CAD build for the part. Positions are in the model's coordinates, mm. A direction names the side the tool comes from. Round coordinates to 2 decimals unless told otherwise and drop trailing zeros. Write each loop counter-clockwise with the first axis right and the second up, starting at its lowest first coordinate (ties: lowest second). Pieces come first, ordered by that corner, then holes. Notation, with made-up numbers: (-27, -21.5) - (13, -21.5) arc R17 cw to (13, -6.5) - close; hole circle Ø8 at (27.5, -35.75). An arc over 180 degrees is marked (long way). Use one line per item in the form item = value. Start each with the question number.
Item 1: Band-saw the part on A-A, the plane z = 0. List the corners of the cut face in (x, y) (3 decimals), and give its area (3 significant figures).
Item 2: Band-saw the part on C-C, the plane x = 13.25. List the corners of the cut face in (y, z), and give its area (3 significant figures).
Item 3: Drill centre lines: L1, parallel to Y at x = 4.5, z = 0 (3 decimals); L2, parallel to X at y = -23, z = 6; L3, parallel to Z at x = 8.75, y = -6. Where is each one in solid material? Low to high.
Item 4: Pull direction Z, two halves, no side cores. Call faces 4 (the flat face through (14, -3, -3)), 5 (the flat face through (11.5, -3, -3)), 6 (the cylindrical face through (12.768, -3.905, 0.867)), 7 (the cylindrical face through (8.93, -6.32, -15.24)): +Z half, -Z half, draft (parallel to the pull), parting line (faces both ways), or undercut.
Item 5: Band-saw the part on D-D, the plane x = 6.25. List the corners of the cut face in (y, z) (3 decimals), and give its area (3 significant figures).
Item 6: Tool access for faces 1 (the cylindrical face through (1.26, 13.24, 13.35)), 2 (the flat face through (4, 0, 17)), 3 (the cylindrical face through (5.67, 3.94, 12.52)): list every direction of +Z, -Z, +X, -X, +Y, -Y with a clear straight run to the whole face (end or side of a thin tool).
Item 7: Pin check, flat tips, straight feed: pin 1 (4.5 mm diameter, centred on y = -14.5, z = -14.5, fed in from +X); pin 2 (5 mm diameter, centred on x = 11, y = -9, fed in from +Z); pin 3 (2 mm diameter, centred on x = 9.5, y = 13, fed in from -Z). Stop position of each tip, or through.
Item 8: Band-saw the part on B-B, the plane y = 0. List the corners of the cut face in (x, z) (3 decimals).
from build123d import *

# Parameters (mm, degrees)
SKETCH1_R                                       = 25
BOSS_EXTRUDE1_DEPTH                             = 4
SKETCH2_R                                       = 16.5
BOSS_EXTRUDE2_DEPTH                             = 10
SKETCH3_R                                       = 12.5
CUT_EXTRUDE1_DEPTH                              = 11.5
SKETCH4_R                                       = 4
CUT_EXTRUDE2_DEPTH                              = 4
M3_CLEARANCE_HOLE1_D                            = 3.4
M3_CLEARANCE_HOLE1_DEPTH                        = 10
CSK_FOR_M3_FLAT_HEAD_MACHINE_SCREW1_D           = 3.4
CSK_FOR_M3_FLAT_HEAD_MACHINE_SCREW1_CSINK_D     = 6.3
CSK_FOR_M3_FLAT_HEAD_MACHINE_SCREW1_CSINK_ANGLE = 90
CIRPATTERN1_COUNT                               = 4
SKETCH10_R                                      = 13.125
CUT_EXTRUDE3_DEPTH                              = 11.5


with BuildPart() as part:
    # Sketch1 → Boss-Extrude1 (new body)
    with BuildSketch(Plane(origin=(0, 0, 0), x_dir=(0, 0, -1), z_dir=(1, 0, 0))):
        Circle(SKETCH1_R)
    extrude(amount=BOSS_EXTRUDE1_DEPTH)

    # Sketch2 → Boss-Extrude2 (add)
    with BuildSketch(Plane(origin=(4, 0, 0), x_dir=(0, 0, -1), z_dir=(1, 0, 0))):
        Circle(SKETCH2_R)
    extrude(amount=BOSS_EXTRUDE2_DEPTH)

    # Sketch3 → Cut-Extrude1 (cut)
    with BuildSketch(Plane.ZY):
        Circle(SKETCH3_R)
    extrude(amount=-CUT_EXTRUDE1_DEPTH, mode=Mode.SUBTRACT)

    # Sketch4 → Cut-Extrude2 (cut)
    with BuildSketch(Plane(origin=(14, 0, 0), x_dir=(0, 0, -1), z_dir=(1, 0, 0))):
        Circle(SKETCH4_R)
    extrude(amount=-CUT_EXTRUDE2_DEPTH, mode=Mode.SUBTRACT)

    # M3 Clearance Hole1
    with Locations(Plane(origin=(14, 0, 0), x_dir=(0, 0, -1), z_dir=(1, 0, 0))):
        with Locations((8.5, 0), (-8.5, 0)):
            Hole(M3_CLEARANCE_HOLE1_D / 2, depth=M3_CLEARANCE_HOLE1_DEPTH)

    # CSK for M3 Flat Head Machine Screw1 (through all)
    with Locations(Plane(origin=(4, 0, 0), x_dir=(0, 0, -1), z_dir=(1, 0, 0))):
        with Locations((-14.495689014, -14.495689014)):
            csk_for_m3_flat_head_machine_screw1 = CounterSinkHole(CSK_FOR_M3_FLAT_HEAD_MACHINE_SCREW1_D / 2, CSK_FOR_M3_FLAT_HEAD_MACHINE_SCREW1_CSINK_D / 2, counter_sink_angle=CSK_FOR_M3_FLAT_HEAD_MACHINE_SCREW1_CSINK_ANGLE)

    # CirPattern1: CSK for M3 Flat Head Machine Screw1 ×4 about axis
    cirpattern1_axis = Axis((0, 0, 0), (1, 0, 0))
    for i in range(1, CIRPATTERN1_COUNT):
        add(csk_for_m3_flat_head_machine_screw1.rotate(cirpattern1_axis, i * 360 / CIRPATTERN1_COUNT), mode=Mode.SUBTRACT)

    # Sketch10 → Cut-Extrude3 (cut)
    with BuildSketch(Plane.ZY):
        Circle(SKETCH10_R)
    extrude(amount=-CUT_EXTRUDE3_DEPTH, mode=Mode.SUBTRACT)


solid = part.part
Determined:
q1.outline = (0, -25) - (4, -25) - (4, -16.5) - (14, -16.5) - (14, -4) - (11.5, -4) - (11.5, -13.125) - (0, -13.125) - close; (0, 13.125) - (11.5, 13.125) - (11.5, 4) - (14, 4) - (14, 16.5) - (4, 16.5) - (4, 25) - (0, 25) - close
q1.area = 208 mm²
q2.outline = circle Ø33 at (0, 0); hole circle Ø8 at (0, 0); hole circle Ø3.4 at (0, -8.5); hole circle Ø3.4 at (0, 8.5)
q2.area = 787 mm²
q3.L1 = -16.5 to -13.125, 13.125 to 16.5
q3.L2 = 0 to 4
q3.L3 = -15.37 to -11.67, 11.67 to 15.37
q4.face_4 = draft
q4.face_5 = undercut
q4.face_6 = undercut
q4.face_7 = parting line
q5.outline = circle Ø33 at (0, 0); hole circle Ø26.25 at (0, 0)
q5.area = 314 mm²
q6.face_1 = +X, -X
q6.face_2 = +X
q6.face_3 = -X
q7.pin_1 = 3.11
q7.pin_2 = 15.17
q7.pin_3 = -11.32
q8.outline = (0, -25) - (4, -25) - (4, -16.5) - (14, -16.5) - (14, -10.2) - (11.5, -10.2) - (11.5, -13.125) - (0, -13.125) - close; (0, 13.125) - (11.5, 13.125) - (11.5, 10.2) - (14, 10.2) - (14, 16.5) - (4, 16.5) - (4, 25) - (0, 25) - close; (11.5, -6.8) - (14, -6.8) - (14, -4) - (11.5, -4) - close; (11.5, 4) - (14, 4) - (14, 6.8) - (11.5, 6.8) - close
